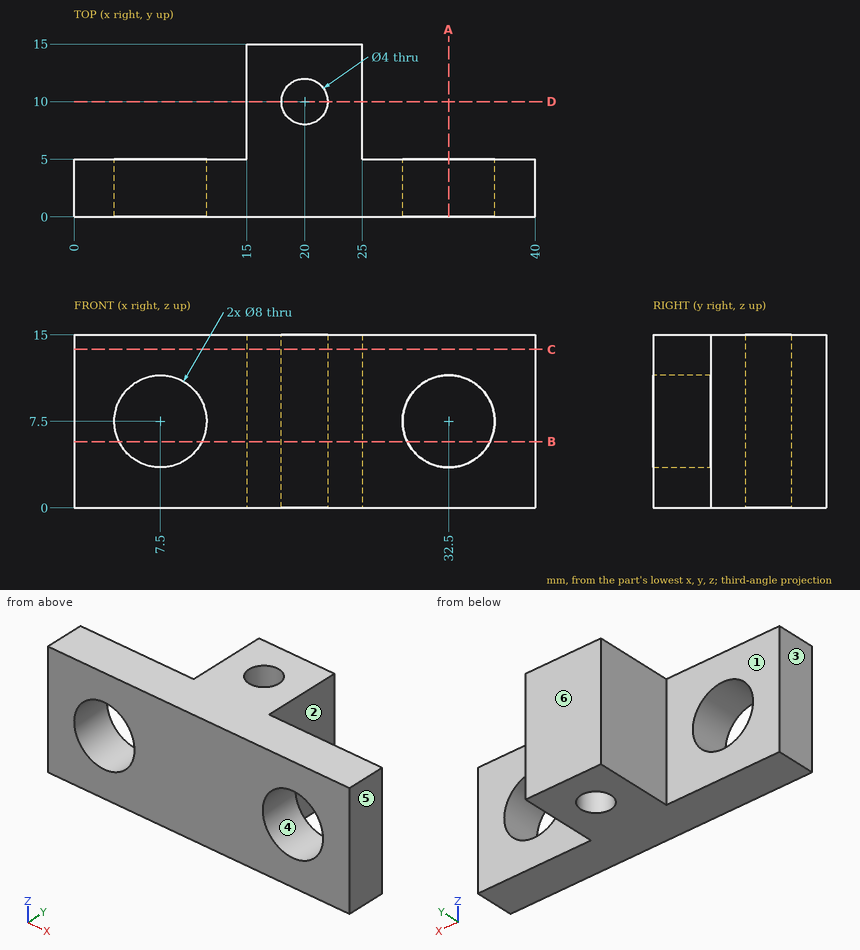
Input: dimensioned drawing with shaded views. Units: mm. Origin: part minimum x, y, z. A direction names the side the tool comes from. Coordinates: 2 decimals unless noted, no trailing zeros. Loops run counter-clockwise (first coordinate to the right, second up) from the corner with the lowest first, then second, coordinate; pieces in that order, holes last. Notation, with made-up numbers: M 79.5,-3 L 138.5,-3 A21 ccw 138.5,9 Z; hole C 71,-24 d2. An arc over 180 degrees is marked long. Use a Markdown table: item, result. Add a question column.
Q1. Section query A-A, the plane x = 32.5. Return loops of the section in (y, z), and give its area (3 significant figures).
Q2. First-contact query: pin 1 (5 mm diameter, centred on y = 12, z = 7, fed in from -X); pin 2 (7.5 mm diameter, centred on x = 6, z = 11, fed in from +Y); pin 3 (3 mm diameter, centred on y = 10.5, z = 11, fed in from +X). Flat tips, straight axial feed; report the tip coordinate or a pass-through.
Q3. Material intervals for L1, parallel to X at y = 1.75, z = 7.5; L2, parallel to Y at x = 20, z = 6.5; L3, parallel to X at y = 14.25, z = 3.25, sorted ascending.
Q4. Draft query along X for the marked faces 4, 5 and 6. Return one class per face: pulls with the +X half, pulls with the -X half, needs draft (parallel to the pull), parting line crosses it, or undercut.
Q5. Section query C-C, the plane z = 13.75. Return loops of the section in (x, y).
Q6. Section query B-B, the plane z = 5.75. Return loops of the section in (x, y).
Q7. Access query for the marked faces 1, 2 and 3. Directions: +Z, -Z, +X, -X, +Y, -Y. A direction counts if a zero-diameter tool reaches every point of the face in a straight line with its end or side. Return the directions, or none.
Q8. Section query D-D, the plane y = 10. Return loops of the section in (x, z).
Result:
| question | item | result |
|---|---|---|
| 1 | outline | M 0,0 L 5,0 L 5,3.5 L 0,3.5 Z; M 0,11.5 L 5,11.5 L 5,15 L 0,15 Z |
| 1 | area | 35.0 mm2 |
| 2 | pin 1 | stops at x = 15 |
| 2 | pin 2 | stops at y = 5 |
| 2 | pin 3 | stops at x = 25 |
| 3 | L1 | x = 0 to 3.5, 11.5 to 28.5, 36.5 to 40 |
| 3 | L2 | y = 0 to 8, 12 to 15 |
| 3 | L3 | x = 15 to 25 |
| 4 | face 4 | undercut |
| 4 | face 5 | pulls with the +X half |
| 4 | face 6 | needs draft |
| 5 | outline | M 0,0 L 40,0 L 40,5 L 25,5 L 25,15 L 15,15 L 15,5 L 0,5 Z; hole C 20,10 d4 |
| 6 | outline | M 0,0 L 3.9,0 L 3.9,5 L 0,5 Z; M 11.1,0 L 28.9,0 L 28.9,5 L 25,5 L 25,15 L 15,15 L 15,5 L 11.1,5 Z; M 36.1,0 L 40,0 L 40,5 L 36.1,5 Z; hole C 20,10 d4 |
| 7 | face 1 | +Z, -Z, -X, +Y |
| 7 | face 2 | +Z, -Z, +X, +Y |
| 7 | face 3 | +Z, -Z, -X, +Y, -Y |
| 8 | outline | M 15,0 L 18,0 L 18,15 L 15,15 Z; M 22,0 L 25,0 L 25,15 L 22,15 Z |
